Build history of the part. All positions in model axes, mm. Give positions to 0.01 mm unless a question says otherwise; leave off trailing zeros. Order: outer loops, then holes, each group sorted by start corner. A loop starts at its lowest first (then second) coordinate and runs counter-clockwise, first axis right, second up. Notation, with made-up numbers: (-18.5, 38) - (-12.5, 38) arc R32 cw to (-12.5, 64) - close; hole circle Ø1 at (-28.75, 70). An arc over 180 degrees is marked (long way). One line per item, written item: value.
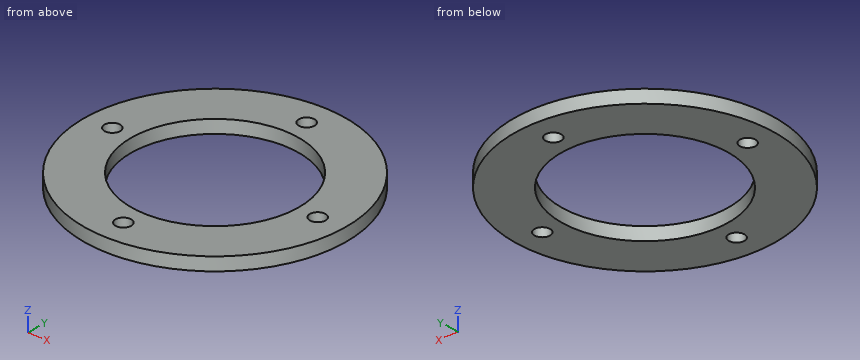
```python
from build123d import *

# Parameters (mm, degrees)
SZKIC1_R                    = 50
DODANIE_WYCI_GNI_CIE1_DEPTH = 5
SZKIC2_R                    = 32
WYTNIJ_WYCI_GNI_CIE1_DEPTH  = 5
SZKIC3_R                    = 3
WYTNIJ_WYCI_GNI_CIE2_DEPTH  = 5


with BuildPart() as part:
    # Szkic1 → Dodanie-wyciągnięcie1 (new body)
    with BuildSketch(Plane.XY):
        Circle(SZKIC1_R)
    extrude(amount=DODANIE_WYCI_GNI_CIE1_DEPTH)

    # Szkic2 → Wytnij-wyciągnięcie1 (cut)
    with BuildSketch(Plane.XY.offset(5)):
        Circle(SZKIC2_R)
    extrude(amount=-WYTNIJ_WYCI_GNI_CIE1_DEPTH, mode=Mode.SUBTRACT)

    # Szkic3 → Wytnij-wyciągnięcie2 (cut)
    with BuildSketch(Plane.XY.offset(5)):
        with Locations((0, 40)):
            Circle(SZKIC3_R)
        with Locations((40, 0)):
            Circle(SZKIC3_R)
        with Locations((0, -40)):
            Circle(SZKIC3_R)
        with Locations((-40, 0)):
            Circle(SZKIC3_R)
    extrude(amount=-WYTNIJ_WYCI_GNI_CIE2_DEPTH, mode=Mode.SUBTRACT)


solid = part.part
```
(1) Slice it at A-A, the plane y = 0. Give the cut face in (x, z).
Completed:
outline: (-50, 0) - (-43, 0) - (-43, 5) - (-50, 5) - close; (-37, 0) - (-32, 0) - (-32, 5) - (-37, 5) - close; (32, 0) - (37, 0) - (37, 5) - (32, 5) - close; (43, 0) - (50, 0) - (50, 5) - (43, 5) - close
(2) Drill centre lines: line 1 (Y direction, x = 0, z = 1.55); line 2 (Y direction, x = -25.5, z = 1.1); line 3 (Y direction, x = -20, z = 3.35). Where is each one in solid material? Low to high.
Completed:
line 1: -50 to -43, -37 to -32, 32 to 37, 43 to 50
line 2: -43.01 to -19.33, 19.33 to 43.01
line 3: -45.83 to -24.98, 24.98 to 45.83
(3) Slice it at B-B, the plane x = -40. Give the cut face in (y, z), and give its area (3 significant figures).
Completed:
outline: (-30, 0) - (-3, 0) - (-3, 5) - (-30, 5) - close; (3, 0) - (30, 0) - (30, 5) - (3, 5) - close
area: 270 mm²
(4) Pin check, flat tips, straight feed: P1, Ø7, axis at x = -40, y = 0, coming from the +Z side; P2, Ø1, axis at x = 9.5, z = 3.5, coming from the -Y side; P3, Ø1.5, axis at y = -37, z = 2.5, coming from the -X side. Stop position of each tip, or through.
Completed:
P1: z = 5
P2: y = -49.18
P3: x = -34.44
